Geometry check sheet. Reference: the model listing, model coordinates, mm. A direction names the side the tool comes from. Give positions to 0.01 mm unless a question says otherwise; leave off trailing zeros. Order: outer loops, then holes, each group sorted by start corner. A loop starts at its lowest first (then second) coordinate and runs counter-clockwise, first axis right, second up. Notation, with made-up numbers: M 74,-3.75 L 78,-3.75 A21 cw 78,13.25 Z; hole C 7,87.25 d7. An arc over 180 degrees is marked long. Answer as CSV lines item,"result".
Autodesk Inventor part; units mm, degrees
ref_plane "Work Plane1" through (-15.24, 0, 3.175) normal (1, 0, 0) x (0, 1, 0)
ref_plane "YZ Plane" through (0, 0, 0) normal (1, 0, 0) x (0, 1, 0)
ref_plane "XZ Plane" through (0, 0, 0) normal (0, 1, 0) x (-1, 0, 0)
sketch "Sketch1" plane through (0, 0, 0) normal (0, 0, 1) x (1, 0, 0)
  circle A0 centre (0, 0) radius 15.24
extrude "Extrusion1" add sketch "Sketch1" along normal blind 3.175
sketch "Sketch2" plane through (0, 0, 3.175) normal (0, 0, 1) x (1, 0, 0)
  circle A0 centre (0, 0) radius 15.24
  line L0 (-15.24, 0) -> (-15.24, 3.175)
  line L1 (-15.24, 0) -> (-15.24, -3.175)
  dimension "d3" = 3.175
  dimension "d4" = 3.175
ref_plane "Work Plane1" through (-15.24, 0, 3.175) normal (1, 0, 0) x (0, 1, 0)
sketch "Sketch3" plane through (-15.24, 0, 3.175) normal (1, 0, 0) x (0, 1, 0)
  line L0 (15.24, 0) -> (-15.24, 0)
  line L1 (-15.24, -3.175) -> (15.24, -3.175)
  line L2 (0, -3.175) -> (3.175, -3.175)
  line L3 (3.175, -3.175) -> (3.175, 0)
  line L4 (3.175, 0) -> (-3.175, 0)
  line L5 (-3.175, 0) -> (-3.175, -3.175)
  line L6 (-3.175, -3.175) -> (3.175, -3.175)
  dimension "d6" = 6.35
extrude "Extrusion2" add sketch "Sketch3" against normal blind 64.2493
sketch "Sketch4" plane through (-15.24, 0, 3.175) normal (1, 0, 0) x (0, 0, -1)
  line L0 (3.175, -3.175) -> (3.175, 0)
  line L1 (0, 3.175) -> (3.175, 3.175)
  line L2 (3.175, 3.175) -> (3.175, -3.175)
  line L3 (3.175, -3.175) -> (0, -3.175)
  line L4 (0, -3.175) -> (0, 3.175)
extrude "Extrusion3" add sketch "Sketch4" along normal blind 12.7
sketch "Sketch6" plane through (0, 0, 0) normal (0, 0, -1) x (-1, 0, 0)
  circle A0 centre (0, 0) radius 3.2385
  dimension "d24" = 6.477
hole "Hole1" at (0, 0, 0) direction (0, 0, -1) diameter 6.477 end through all
hole "Hole2" at (0, 0, 0) direction (0, 0, 1) diameter 6.477 depth 7.9375 tip angle 118
sketch "Sketch7" plane through (0, 0, 3.175) normal (0, 0, 1) x (1, 0, 0)
  line L0 (-79.4893, -3.175) -> (-79.4893, 3.175)
  line L1 (-79.4893, 0) -> (-76.3143, 0)
  circle A0 centre (-76.3143, 0) radius 1.5875
  point P0 (0, 0)
  dimension "d39" = 3.175
  dimension "d40" = 3.175
extrude "Extrusion6" cut sketch "Sketch7" against normal blind 25.4
sketch "Sketch8" plane through (0, 0, 3.175) normal (0, 0, 1) x (1, 0, 0)
  arc A0 (-14.9056, -3.175) -> (-14.9056, 3.175) centre (0, 0) ccw
  line L0 (-32.1247, -25.4) -> (18.6753, -25.4)
  line L1 (-32.1247, -25.4) -> (-82.9246, -25.4)
  line L2 (-32.1247, 25.4) -> (-82.9246, 25.4)
  line L3 (-32.1247, 25.4) -> (18.6753, 25.4)
  line L4 (18.6753, 25.4) -> (18.6753, -25.4)
  line L5 (-82.9246, 25.4) -> (-82.9246, -25.4)
  dimension "d45" = 50.8
  dimension "d46" = 50.8
  dimension "d47" = 50.8
  dimension "d48" = 50.8
extrude "Extrusion7" add sketch "Sketch8" along normal blind 3.175
sketch "Sketch9" plane through (-79.4893, -3.175, 0) normal (0, -1, 0) x (1, 0, 0)
  line L0 (64.5837, 3.175) -> (64.5837, 0)
  line L1 (64.5837, 0) -> (64.5837, 3.175)
  point P0 (79.4893, 0)
sketch "Sketch10" plane through (-79.4893, 3.175, 0) normal (0, 1, 0) x (1, 0, 0)
  line L0 (64.5837, -3.175) -> (64.5837, 0)
  line L1 (64.5837, 0) -> (64.5837, -3.175)
  point P0 (79.4893, 0)
sketch "Sketch11" plane through (0, 0, 3.175) normal (0, 0, -1) x (-1, 0, 0)
  line L0 (14.9056, 3.175) -> (79.4893, 3.175)
  line L1 (79.4893, 3.175) -> (79.4893, -3.175)
  line L2 (14.9056, 3.175) -> (79.4893, 3.175)
  line L3 (79.4893, -3.175) -> (14.9056, -3.175)
  line L4 (14.9056, -3.175) -> (79.4893, -3.175)
  arc A0 (14.9056, 3.175) -> (14.9056, -3.175) centre (0, 0) ccw
  circle A1 centre (0, 0) radius 3.2385
  line L5 (79.4893, -3.175) -> (14.9056, -3.175)
  dimension "d51" = 64.5837
  dimension "d52" = 64.5837
  dimension "d53" = 18.4785
  dimension "d54" = 6.35
  dimension "d55" = 14.9056
sketch "Sketch12" plane through (-82.9246, -25.4, 3.175) normal (0, -1, 0) x (1, 0, 0)
  line L0 (0, 0) -> (101.6, 0)
  line L1 (68.019, -3.175) -> (98.1646, -3.175)
  point P0 (82.9246, -3.175)
  dimension "d56" = 3.175
sketch "Sketch13" plane through (0, 0, 3.175) normal (0, 0, -1) x (-1, 0, 0)
  point P0 (0, 0)
sketch "Sketch14" plane through (0, 0, 0) normal (0, 0, -1) x (-1, 0, 0)
  circle A0 centre (0, 0) radius 15.24
  circle A1 centre (76.3143, 0) radius 1.5875
  circle A2 centre (0, 0) radius 3.2385
  line L0 (79.4893, -3.175) -> (14.9056, -3.175)
  line L1 (79.4893, 3.175) -> (79.4893, -3.175)
  line L2 (14.9056, 3.175) -> (79.4893, 3.175)
  arc A3 (14.9056, 3.175) -> (14.9056, -3.175) centre (0, 0) ccw
  line L3 (15.24, -15.24) -> (15.24, 15.24)
  line L4 (-18.6753, 25.4) -> (82.9246, 25.4)
  line L5 (-18.6753, -25.4) -> (-18.6753, 25.4)
  line L6 (82.9246, -25.4) -> (-18.6753, -25.4)
  line L7 (82.9246, 25.4) -> (82.9246, -25.4)
  line L8 (79.4893, 3.175) -> (14.9056, 3.175)
  line L9 (79.4893, -3.175) -> (79.4893, 3.175)
  line L10 (79.4893, -3.175) -> (14.9056, -3.175)
  arc A4 (14.9056, 3.175) -> (14.9056, -3.175) centre (0, 0) ccw
  line L11 (14.9056, -3.175) -> (14.9056, -3.5133)
  dimension "d57" = 0.3344
properties part number "ClawLinkage"
(1) Draft check along X on faces 6 (the face through (-77.9, 0.1, 1.6)), 7 (the face through (-12, 0, 0)), 8 (the face through (18.675, 0, 5)). Enter one of: +X half, -X half, draft (parallel to the pull), parting line (faces both ways), or undercut.
The answers:
face 6,"undercut"
face 7,"draft"
face 8,"+X half"
(2) Tool access check on faces 1 (the face through (-79.489, 0, 2)), 2 (the face through (-48, -3.175, 2)), 3 (the face through (15.227, 0.625, 1.565)), 4 (the face through (-47, 3.175, 2)), 5 (the face through (-31, 25.4, 5)). Record the directions out of +Z, -Z, +X, -X, +Y, -Y that give a thin tool (end or side, any length) a straight path to the whole face; none if there is none.
The answers:
face 1,"-Z, -X, +Y, -Y"
face 2,"-Z, -X, -Y"
face 3,"-Z"
face 4,"-Z, -X, +Y"
face 5,"+Z, -Z, +X, -X, +Y"
(3) Section check D-D on x = -16.5. Enter the section's corners in (y, z) (3 decimals), then the cut area to 3 significant figures.
The answers:
outline,"M -25.4,3.175 L -3.175,3.175 L -3.175,0 L 3.175,0 L 3.175,3.175 L 25.4,3.175 L 25.4,6.35 L -25.4,6.35 Z"
area,"181 mm2"
(4) Gauge pin test, flat ends, axial feed: P1, Ø3.5, axis at y = -0.5, z = 2, coming from the -X side; P2, Ø1, axis at x = -55.5, z = 1.5, coming from the +Y side (3 decimals); P3, Ø1.6, axis at x = -56, z = 1, coming from the -Y side (3 decimals); P4, Ø4, axis at x = 0, y = 0, coming from the -Z side (3 decimals). Record the tip position at first contact, or that the pin passes through.
The answers:
P1,"stops at x = -82.92"
P2,"stops at y = 3.175"
P3,"stops at y = -3.175"
P4,"stops at z = 3.175"
(5) Section check B-B on z = 1. Enter the section's corners in (x, y) (1 decimal), then the cut area to 3 significant figures.
The answers:
outline,"M -79.5,-3.2 L -14.9,-3.2 A15.2 ccw long -14.9,3.2 L -79.5,3.2 Z; hole C -76.3,0 d3.2; hole C 0,0 d6.5"
area,"1,100 mm2"
(6) Material ranges on line 1 (X direction, y = 0, z = 1.25); line 2 (Y direction, x = 0, z = 1.95); line 3 (Z direction, x = -35, y = 7) (3 decimals), recorded low to high.
The answers:
line 1,"x = -79.49 to -77.9, -74.73 to -3.24, 3.24 to 15.24"
line 2,"y = -15.24 to -3.24, 3.24 to 15.24"
line 3,"z = 3.175 to 6.35"
